Here's the drawing with two shaded views (mm, measured from the low corner). I have some questions. Round coordinates to 2 decimals unless told otherwise and drop trailing zeros. Write each loop counter-clockwise with the first axis right and the second up, starting at its lowest first coordinate (ties: lowest second). Pieces come first, ordered by that corner, then holes. Notation, with made-up numbers: (19, 42) -> (54, 42) arc R37 cw to (54, 81) -> close; hole circle Ø7 at (9.25, -16). An arc over 180 degrees is marked (long way). Use CSV: the item, a comma, the result in double quotes.
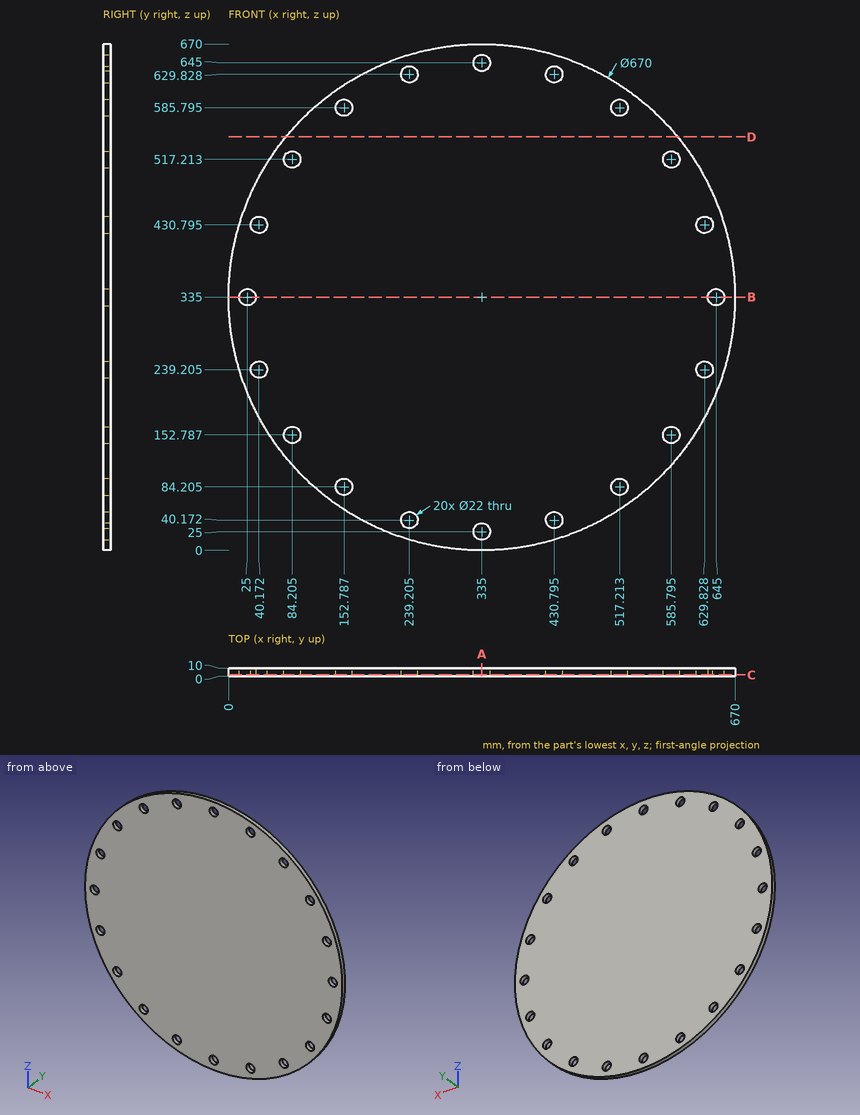
Q1. Suppose I cut it at D-D (z = 547). Write out the boundary of the cut face in (x, y) (1 decimal), and give its area (3 significant figures).
Resolved:
outline,"(75.6, 0) -> (594.4, 0) -> (594.4, 10) -> (75.6, 10) -> close"
area,"5,190 mm^2"
Q2. Please list where these lines run through material, in increasing order: probe 1 along Z at (x, y) = (325.5, 8) (1 decimal); probe 2 along Z at (x, y) = (93.5, 5.5) (1 decimal); probe 3 along X at (y, z) = (4, 507) (1 decimal).
Resolved:
probe 1,"z = 0.1 to 19.5, 30.5 to 639.5, 650.5 to 669.9"
probe 2,"z = 102.8 to 146.9, 158.7 to 511.3, 523.1 to 567.2"
probe 3,"x = 47.5 to 80.1, 88.3 to 581.7, 589.9 to 622.5"
Q3. Will these pins go through, and if not, where does the flat tip stop? P1, Ø17.5, axis at x = 629.83, z = 430.8, coming from the -Y side; P2, Ø4, axis at x = 352.5, y = 8, coming from the -Z side; P3, Ø4, axis at x = 286.5, y = 8, coming from the -Z side; P4, Ø5, axis at y = 4, z = 229.5, coming from the +X side.
Resolved:
P1,"passes through"
P2,"stops at z = 0.36"
P3,"stops at z = 3.24"
P4,"stops at x = 653.77"
Q4. Suppose I cut it at A-A (x = 335). Write out the boundary of the cut face in (y, z), and give its area (3 significant figures).
Resolved:
outline,"(0, 0) -> (10, 0) -> (10, 14) -> (0, 14) -> close; (0, 36) -> (10, 36) -> (10, 634) -> (0, 634) -> close; (0, 656) -> (10, 656) -> (10, 670) -> (0, 670) -> close"
area,"6,260 mm^2"
Q5. Suppose I cut it at C-C (y = 1.5). Count the separate pieces of the cut face and the enclosed holes in it, and give its area (3 significant figures).
Resolved:
separate pieces,"1"
enclosed holes,"20"
area,"345,000 mm^2"
Q6. Suppose I cut it at B-B (z = 335). Write out the boundary of the cut face in (x, y), and give its area (3 significant figures).
Resolved:
outline,"(0, 0) -> (14, 0) -> (14, 10) -> (0, 10) -> close; (36, 0) -> (634, 0) -> (634, 10) -> (36, 10) -> close; (656, 0) -> (670, 0) -> (670, 10) -> (656, 10) -> close"
area,"6,260 mm^2"
